Geometry check sheet. Reference: the model listing, model coordinates, mm. Coordinates: 2 decimals unless noted, no trailing zeros. One line per item, written item: value. Start each with the question number.
```python
from build123d import *

# Parameters (mm, degrees)
F1_DEPTH = 1500
F3_DEPTH = 1500.001
F4_R     = 2.1
F5_DEPTH = 1500.001


with BuildPart() as f1:
    # F0 (on Top) → F1 (new body)
    with BuildSketch(Plane.XY):
        Polygon((0, 5.2), (0, 0), (5.2, 0), (7, 1.8), (4.4, 1.8), (4.4, 3.44), (7.16, 6.2), (12.84, 6.2), (15.6, 3.44), (15.6, 1.8), (13, 1.8), (14.8, 0), (25.2, 0), (27, 1.8), (24.4, 1.8), (24.4, 3.44), (27.16, 6.2), (32.84, 6.2), (35.6, 3.44), (35.6, 1.8), (33, 1.8), (34.8, 0), (40, 0), (40, 5.2), (38.2, 7), (38.2, 4.4), (36.56, 4.4), (33.8, 7.16), (33.8, 12.84), (36.56, 15.6), (38.2, 15.6), (38.2, 13), (40, 14.8), (40, 20), (34.8, 20), (33, 18.2), (35.6, 18.2), (35.6, 16.56), (32.84, 13.8), (27.16, 13.8), (24.4, 16.56), (24.4, 18.2), (27, 18.2), (25.2, 20), (14.8, 20), (13, 18.2), (15.6, 18.2), (15.6, 16.56), (12.84, 13.8), (7.16, 13.8), (4.4, 16.56), (4.4, 18.2), (7, 18.2), (5.2, 20), (0, 20), (0, 14.8), (1.8, 13), (1.8, 15.6), (3.44, 15.6), (6.2, 12.84), (6.2, 7.16), (3.44, 4.4), (1.8, 4.4), (1.8, 7), align=None)
    extrude(amount=F1_DEPTH)

    # F2 (on face) → F3 (cut, through all)
    with BuildSketch(Plane.XY.offset(1500)):
        Polygon((3.33, 18.2), (1.8, 18.2), (1.8, 16.67), align=None)
        Polygon((1.8, 3.33), (1.8, 1.8), (3.33, 1.8), align=None)
        Polygon((36.67, 1.8), (38.2, 1.8), (38.2, 3.33), align=None)
        Polygon((38.2, 16.67), (38.2, 18.2), (36.67, 18.2), align=None)
    extrude(amount=-F3_DEPTH, mode=Mode.SUBTRACT)

    # F4 (on face) → F5 (cut, through all)
    with BuildSketch(Plane.XY.offset(1500)):
        Polygon((22.9, 18.2), (17.1, 18.2), (17.1, 16.24), (13.7, 12.84), (13.7, 7.16), (17.1, 3.76), (17.1, 1.8), (22.9, 1.8), (22.9, 3.76), (26.3, 7.16), (26.3, 12.84), (22.9, 16.24), align=None)
        with Locations((30, 10)):
            Circle(F4_R)
        with Locations((10, 10)):
            Circle(F4_R)
    extrude(amount=-F5_DEPTH, mode=Mode.SUBTRACT)


solid = f1.part
```
Q1. Gauge pin test, flat ends, axial feed: P1, Ø1.3, axis at x = 34, z = 999, coming from the -Y side; P2, Ø0.8, axis at x = 26, z = 1086, coming from the +Y side; P3, Ø1.3, axis at y = 6.5, z = 414, coming from the +X side. Record the tip position at first contact, or that the pin passes through.
Q2. Material ranges on probe 1 along Y at (x, z) = (5, 343); probe 2 along X at (y, z) = (10.75, 742.5); probe 3 along X at (y, z) = (19, 1275), recorded low to high.
Q3. Cross-section at A-A, the plane z = 1019. Count the separate pieces of the cut face and the enclosed holes in it, and give its area (3 significant figures).
Check result:
1. P1: stops at y = 0.15
1. P2: stops at y = 19.6
1. P3: stops at x = 39.35
2. probe 1: y = 0 to 1.8, 4.04 to 5.96, 14.04 to 15.96, 18.2 to 20
2. probe 2: x = 6.2 to 8.04, 11.96 to 13.7, 26.3 to 28.04, 31.96 to 33.8
2. probe 3: x = 0 to 6.2, 13.8 to 26.2, 33.8 to 40
3. separate pieces: 1
3. enclosed holes: 7
3. area: 277 mm2
